Verification items for the finished model (mm, model axes). Face numbers are marked on the shaded views. A direction names the side the tool comes from. Round coordinates to 2 decimals unless told otherwise and drop trailing zeros. Order: outer loops, then holes, each group sorted by start corner. A loop starts at its lowest first (then second) coordinate and runs counter-clockwise, first axis right, second up. Notation, with made-up numbers: (73, -3) -> (107, -3) arc R30 cw to (107, 22) -> close; hole circle Ø4 at (13.5, -3). An arc over 180 degrees is marked (long way). Return JSON: item names as keys, results as strings. Group by question number.
1) Section check B-B on z = -10.5. Enter the section's corners in (x, y), plus the area to 3 significant figures.
2) Tool access check on the marked faces 1 and 2. Record the directions out of +Z, -Z, +X, -X, +Y, -Y that give a thin tool (end or side, any length) a straight path to the whole face; none if there is none.
3) Scan lines: L1, parallel to X at y = 1.6, z = -21; L2, parallel to Z at x = 3, y = 0.4; L3, parallel to Y at x = -11.5, z = 31. Record each from-to range of solid material in increasing order.
4) Depth check by flat-ended pin: pin 1 (2.5 mm diameter, centred on x = -20.81, z = -4.15, fed in from +Y); pin 2 (4 mm diameter, centred on x = 5, z = 9.5, fed in from -Y). Enter the tip coordinate at first touch or a pass-through.
5) Section check C-C on y = 0.85. State how many separate pieces and enclosed holes the cut face has, plus the area to 3 significant figures.
6) Section check A-A on x = 33. Enter the section's corners in (y, z), plus the area to 3 significant figures.
```python
from build123d import *

# Parameters (mm, degrees)
SKETCH1_W           = 80
SKETCH1_H           = 80
BOSS_EXTRUDE1_DEPTH = 2
FILLET1_R           = 2
SKETCH3_W           = 70
SKETCH3_H           = 70
CUT_EXTRUDE2_DEPTH  = 0.5
SKETCH4_W           = 70
SKETCH4_H           = 70
CUT_EXTRUDE3_DEPTH  = 0.5
SKETCH5_R           = 1
CUT_EXTRUDE4_DEPTH  = 10


with BuildPart() as part:
    # Sketch1 → Boss-Extrude1 (new body)
    with BuildSketch(Plane(origin=(0, 0, 0), x_dir=(1, 0, 0), z_dir=(0, 1, 0))):
        Rectangle(SKETCH1_W, SKETCH1_H)
    extrude(amount=BOSS_EXTRUDE1_DEPTH)

    # Fillet1
    fillet1_edges = [part.edges().sort_by_distance(p)[0] for p in [
        (-40, 1, -40),
        (40, 1, -40),
        (40, 1, 40),
        (-40, 1, 40),
    ]]
    fillet(fillet1_edges, radius=FILLET1_R)

    # Sketch3 → Cut-Extrude2 (cut)
    with BuildSketch(Plane(origin=(0, 2, 0), x_dir=(1, 0, 0), z_dir=(0, 1, 0))):
        Rectangle(SKETCH3_W, SKETCH3_H)
    extrude(amount=-CUT_EXTRUDE2_DEPTH, mode=Mode.SUBTRACT)

    # Sketch4 → Cut-Extrude3 (cut)
    with BuildSketch(Plane.XZ):
        Rectangle(SKETCH4_W, SKETCH4_H)
    extrude(amount=-CUT_EXTRUDE3_DEPTH, mode=Mode.SUBTRACT)

    # Sketch5 → Cut-Extrude4 (cut)
    with BuildSketch(Plane(origin=(0, 2, 0), x_dir=(1, 0, 0), z_dir=(0, 1, 0))):
        with Locations(Location((37.5, -37.5, 0), (0, 0, 270))):
            Circle(SKETCH5_R)
        with Locations(Location((29.17, -37.5, 0), (0, 0, 270))):
            Circle(SKETCH5_R)
        with Locations(Location((20.84, -37.5, 0), (0, 0, 270))):
            Circle(SKETCH5_R)
        with Locations(Location((12.51, -37.5, 0), (0, 0, 270))):
            Circle(SKETCH5_R)
        with Locations(Location((4.18, -37.5, 0), (0, 0, 270))):
            Circle(SKETCH5_R)
        with Locations(Location((-4.15, -37.5, 0), (0, 0, 270))):
            Circle(SKETCH5_R)
        with Locations(Location((-12.48, -37.5, 0), (0, 0, 270))):
            Circle(SKETCH5_R)
        with Locations(Location((-20.81, -37.5, 0), (0, 0, 270))):
            Circle(SKETCH5_R)
        with Locations(Location((-29.14, -37.5, 0), (0, 0, 270))):
            Circle(SKETCH5_R)
        with Locations(Location((-37.47, -37.5, 0), (0, 0, 270))):
            Circle(SKETCH5_R)
        with Locations(Location((29.17, -29.17, 0), (0, 0, 90))):
            Circle(SKETCH5_R)
        with Locations(Location((20.84, -29.17, 0), (0, 0, 90))):
            Circle(SKETCH5_R)
        with Locations(Location((12.51, -29.17, 0), (0, 0, 90))):
            Circle(SKETCH5_R)
        with Locations(Location((4.18, -29.17, 0), (0, 0, 90))):
            Circle(SKETCH5_R)
        with Locations(Location((-4.15, -29.17, 0), (0, 0, 90))):
            Circle(SKETCH5_R)
        with Locations(Location((-12.48, -29.17, 0), (0, 0, 90))):
            Circle(SKETCH5_R)
        with Locations(Location((-20.81, -29.17, 0), (0, 0, 90))):
            Circle(SKETCH5_R)
        with Locations(Location((-29.14, -29.17, 0), (0, 0, 90))):
            Circle(SKETCH5_R)
        with Locations(Location((-37.47, -29.17, 0), (0, 0, 270))):
            Circle(SKETCH5_R)
        with Locations(Location((29.17, -20.84, 0), (0, 0, 90))):
            Circle(SKETCH5_R)
        with Locations(Location((20.84, -20.84, 0), (0, 0, 90))):
            Circle(SKETCH5_R)
        with Locations(Location((12.51, -20.84, 0), (0, 0, 90))):
            Circle(SKETCH5_R)
        with Locations(Location((4.18, -20.84, 0), (0, 0, 90))):
            Circle(SKETCH5_R)
        with Locations(Location((-4.15, -20.84, 0), (0, 0, 90))):
            Circle(SKETCH5_R)
        with Locations(Location((-12.48, -20.84, 0), (0, 0, 90))):
            Circle(SKETCH5_R)
        with Locations(Location((-20.81, -20.84, 0), (0, 0, 90))):
            Circle(SKETCH5_R)
        with Locations(Location((-29.14, -20.84, 0), (0, 0, 90))):
            Circle(SKETCH5_R)
        with Locations(Location((-37.47, -20.84, 0), (0, 0, 270))):
            Circle(SKETCH5_R)
        with Locations(Location((29.17, -12.51, 0), (0, 0, 90))):
            Circle(SKETCH5_R)
        with Locations(Location((20.84, -12.51, 0), (0, 0, 90))):
            Circle(SKETCH5_R)
        with Locations(Location((12.51, -12.51, 0), (0, 0, 90))):
            Circle(SKETCH5_R)
        with Locations(Location((4.18, -12.51, 0), (0, 0, 90))):
            Circle(SKETCH5_R)
        with Locations(Location((-4.15, -12.51, 0), (0, 0, 90))):
            Circle(SKETCH5_R)
        with Locations(Location((-12.48, -12.51, 0), (0, 0, 90))):
            Circle(SKETCH5_R)
        with Locations(Location((-20.81, -12.51, 0), (0, 0, 90))):
            Circle(SKETCH5_R)
        with Locations(Location((-29.14, -12.51, 0), (0, 0, 90))):
            Circle(SKETCH5_R)
        with Locations(Location((-37.47, -12.51, 0), (0, 0, 270))):
            Circle(SKETCH5_R)
        with Locations(Location((29.17, -4.18, 0), (0, 0, 90))):
            Circle(SKETCH5_R)
        with Locations(Location((20.84, -4.18, 0), (0, 0, 90))):
            Circle(SKETCH5_R)
        with Locations(Location((12.51, -4.18, 0), (0, 0, 90))):
            Circle(SKETCH5_R)
        with Locations(Location((4.18, -4.18, 0), (0, 0, 90))):
            Circle(SKETCH5_R)
        with Locations(Location((-4.15, -4.18, 0), (0, 0, 90))):
            Circle(SKETCH5_R)
        with Locations(Location((-12.48, -4.18, 0), (0, 0, 90))):
            Circle(SKETCH5_R)
        with Locations(Location((-20.81, -4.18, 0), (0, 0, 90))):
            Circle(SKETCH5_R)
        with Locations(Location((-29.14, -4.18, 0), (0, 0, 90))):
            Circle(SKETCH5_R)
        with Locations(Location((-37.47, -4.18, 0), (0, 0, 270))):
            Circle(SKETCH5_R)
        with Locations(Location((29.17, 4.15, 0), (0, 0, 90))):
            Circle(SKETCH5_R)
        with Locations(Location((20.84, 4.15, 0), (0, 0, 90))):
            Circle(SKETCH5_R)
        with Locations(Location((12.51, 4.15, 0), (0, 0, 90))):
            Circle(SKETCH5_R)
        with Locations(Location((4.18, 4.15, 0), (0, 0, 90))):
            Circle(SKETCH5_R)
        with Locations(Location((-4.15, 4.15, 0), (0, 0, 90))):
            Circle(SKETCH5_R)
        with Locations(Location((-12.48, 4.15, 0), (0, 0, 90))):
            Circle(SKETCH5_R)
        with Locations(Location((-20.81, 4.15, 0), (0, 0, 90))):
            Circle(SKETCH5_R)
        with Locations(Location((-29.14, 4.15, 0), (0, 0, 90))):
            Circle(SKETCH5_R)
        with Locations(Location((-37.47, 4.15, 0), (0, 0, 270))):
            Circle(SKETCH5_R)
        with Locations(Location((29.17, 12.48, 0), (0, 0, 90))):
            Circle(SKETCH5_R)
        with Locations(Location((20.84, 12.48, 0), (0, 0, 90))):
            Circle(SKETCH5_R)
        with Locations(Location((12.51, 12.48, 0), (0, 0, 90))):
            Circle(SKETCH5_R)
        with Locations(Location((4.18, 12.48, 0), (0, 0, 90))):
            Circle(SKETCH5_R)
        with Locations(Location((-4.15, 12.48, 0), (0, 0, 90))):
            Circle(SKETCH5_R)
        with Locations(Location((-12.48, 12.48, 0), (0, 0, 90))):
            Circle(SKETCH5_R)
        with Locations(Location((-20.81, 12.48, 0), (0, 0, 90))):
            Circle(SKETCH5_R)
        with Locations(Location((-29.14, 12.48, 0), (0, 0, 90))):
            Circle(SKETCH5_R)
        with Locations(Location((-37.47, 12.48, 0), (0, 0, 270))):
            Circle(SKETCH5_R)
        with Locations(Location((29.17, 20.81, 0), (0, 0, 90))):
            Circle(SKETCH5_R)
        with Locations(Location((20.84, 20.81, 0), (0, 0, 90))):
            Circle(SKETCH5_R)
        with Locations(Location((12.51, 20.81, 0), (0, 0, 90))):
            Circle(SKETCH5_R)
        with Locations(Location((4.18, 20.81, 0), (0, 0, 90))):
            Circle(SKETCH5_R)
        with Locations(Location((-4.15, 20.81, 0), (0, 0, 90))):
            Circle(SKETCH5_R)
        with Locations(Location((-12.48, 20.81, 0), (0, 0, 90))):
            Circle(SKETCH5_R)
        with Locations(Location((-20.81, 20.81, 0), (0, 0, 90))):
            Circle(SKETCH5_R)
        with Locations(Location((-29.14, 20.81, 0), (0, 0, 90))):
            Circle(SKETCH5_R)
        with Locations(Location((-37.47, 20.81, 0), (0, 0, 270))):
            Circle(SKETCH5_R)
        with Locations(Location((29.17, 29.14, 0), (0, 0, 90))):
            Circle(SKETCH5_R)
        with Locations(Location((20.84, 29.14, 0), (0, 0, 90))):
            Circle(SKETCH5_R)
        with Locations(Location((12.51, 29.14, 0), (0, 0, 90))):
            Circle(SKETCH5_R)
        with Locations(Location((4.18, 29.14, 0), (0, 0, 90))):
            Circle(SKETCH5_R)
        with Locations(Location((-4.15, 29.14, 0), (0, 0, 90))):
            Circle(SKETCH5_R)
        with Locations(Location((-12.48, 29.14, 0), (0, 0, 90))):
            Circle(SKETCH5_R)
        with Locations(Location((-20.81, 29.14, 0), (0, 0, 90))):
            Circle(SKETCH5_R)
        with Locations(Location((-29.14, 29.14, 0), (0, 0, 90))):
            Circle(SKETCH5_R)
        with Locations(Location((-37.47, 29.14, 0), (0, 0, 270))):
            Circle(SKETCH5_R)
        with Locations(Location((29.17, 37.47, 0), (0, 0, 270))):
            Circle(SKETCH5_R)
        with Locations(Location((20.84, 37.47, 0), (0, 0, 270))):
            Circle(SKETCH5_R)
        with Locations(Location((12.51, 37.47, 0), (0, 0, 270))):
            Circle(SKETCH5_R)
        with Locations(Location((4.18, 37.47, 0), (0, 0, 270))):
            Circle(SKETCH5_R)
        with Locations(Location((-4.15, 37.47, 0), (0, 0, 270))):
            Circle(SKETCH5_R)
        with Locations(Location((-12.48, 37.47, 0), (0, 0, 270))):
            Circle(SKETCH5_R)
        with Locations(Location((-20.81, 37.47, 0), (0, 0, 270))):
            Circle(SKETCH5_R)
        with Locations(Location((-29.14, 37.47, 0), (0, 0, 270))):
            Circle(SKETCH5_R)
        with Locations(Location((-37.47, 37.47, 0), (0, 0, 270))):
            Circle(SKETCH5_R)
        with Locations(Location((37.5, -29.17, 0), (0, 0, 270))):
            Circle(SKETCH5_R)
        with Locations(Location((37.5, -20.84, 0), (0, 0, 270))):
            Circle(SKETCH5_R)
        with Locations(Location((37.5, -12.51, 0), (0, 0, 270))):
            Circle(SKETCH5_R)
        with Locations(Location((37.5, -4.18, 0), (0, 0, 270))):
            Circle(SKETCH5_R)
        with Locations(Location((37.5, 4.15, 0), (0, 0, 270))):
            Circle(SKETCH5_R)
        with Locations(Location((37.5, 12.48, 0), (0, 0, 270))):
            Circle(SKETCH5_R)
        with Locations(Location((37.5, 20.81, 0), (0, 0, 270))):
            Circle(SKETCH5_R)
        with Locations(Location((37.5, 29.14, 0), (0, 0, 270))):
            Circle(SKETCH5_R)
        with Locations(Location((37.5, 37.47, 0), (0, 0, 270))):
            Circle(SKETCH5_R)
    extrude(amount=-CUT_EXTRUDE4_DEPTH, mode=Mode.SUBTRACT)


solid = part.part
```
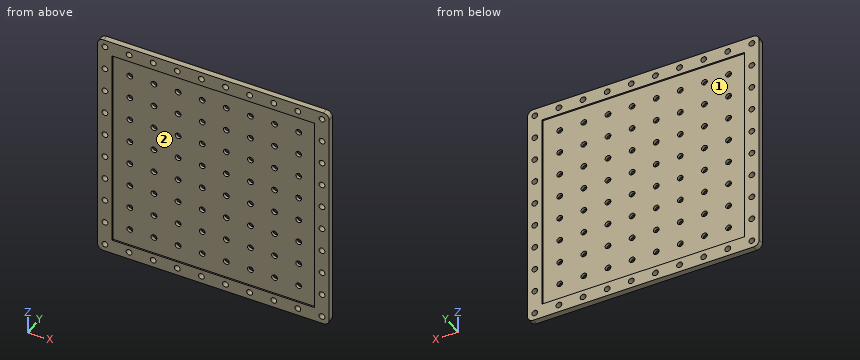
Check result:
{
 "1": {"outline": "(-40, 0) -> (-35, 0) -> (-35, 0.5) -> (35, 0.5) -> (35, 0) -> (40, 0) -> (40, 2) -> (35, 2) -> (35, 1.5) -> (-35, 1.5) -> (-35, 2) -> (-40, 2) -> close", "area": "90.0 mm^2"},
 "2": {"face 1": "+Y", "face 2": "-Y"},
 "3": {"L1": "-40 to -38.45, -36.49 to -35, 35 to 36.52, 38.48 to 40", "L2": "-40 to -35, 35 to 40", "L3": "0.5 to 1.5"},
 "4": {"pin 1": "y = 1.5", "pin 2": "y = 0.5"},
 "5": {"separate pieces": "1", "enclosed holes": "100", "area": "6,080 mm^2"},
 "6": {"outline": "(0, -40) -> (2, -40) -> (2, -35) -> (1.5, -35) -> (1.5, 35) -> (2, 35) -> (2, 40) -> (0, 40) -> (0, 35) -> (0.5, 35) -> (0.5, -35) -> (0, -35) -> close", "area": "90.0 mm^2"}
}
